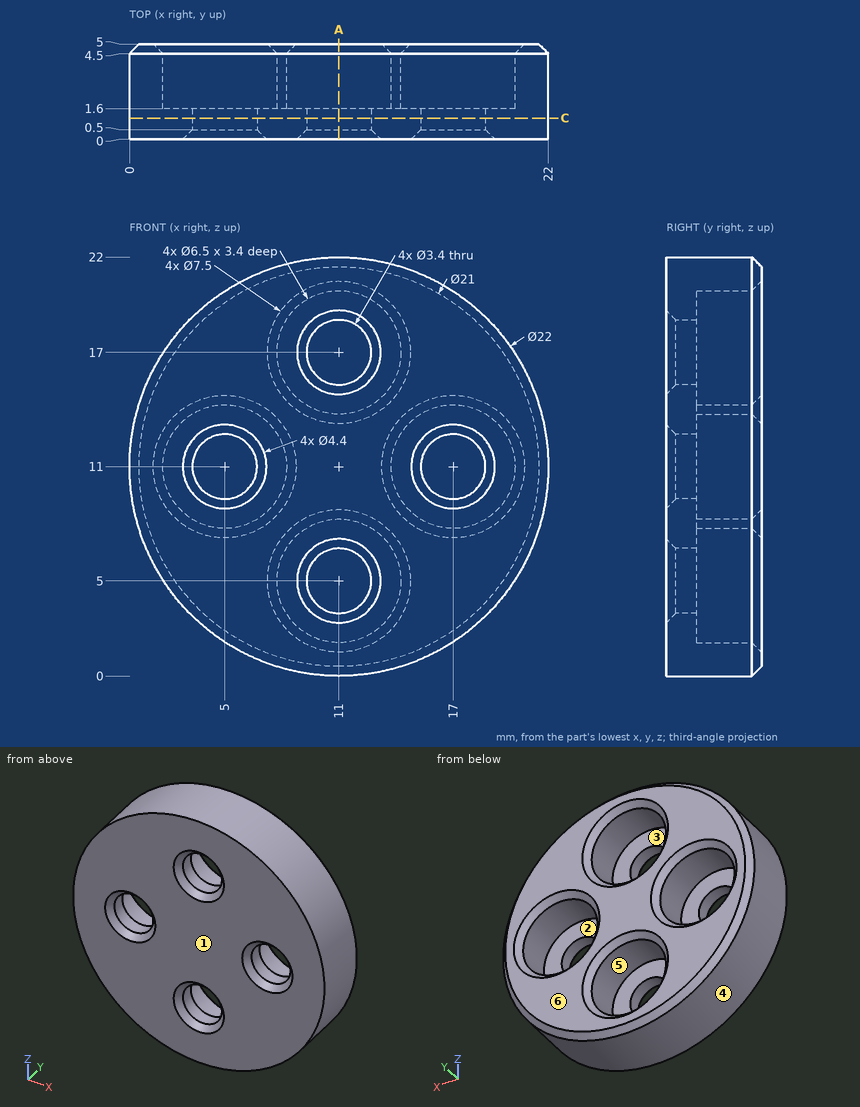
Check sheet for the drawn part. Datum: minimum x, y, z corner. Units: mm. A direction names the side the tool comes from. Give positions to 0.01 mm unless a question says otherwise; leave off trailing zeros. Write each loop counter-clockwise with the first axis right and the second up, starting at its lowest first coordinate (ties: lowest second). Pieces come first, ordered by that corner, then holes.
(1) Gauge pin test, flat ends, axial feed: pin 1 (6 mm diameter, centred on x = 11, z = 17, fed in from -Y); pin 2 (2.5 mm diameter, centred on x = 11, z = 17, fed in from -Y); pin 3 (4 mm diameter, centred on x = 11, z = 5, fed in from +Y); pin 4 (3 mm diameter, centred on y = 4, z = 16.5, fed in from +X). Record the tip position at first contact, or that the pin passes through.
(2) Cross-section at A-A (x = 11). State how many separate pieces and enclosed holes the cut face has, plus the area to 3 significant figures.
(3) Access from +Z, -Z, +X, -X, +Y, -Y to the whole of each face (thin tool, end or side, straight path). Record for the marked faces 5 and 6.
(4) Mould release check, pull along X, two halves, no side actions. Record for the marked faces 1, 2, 3 and 4: +X half, -X half, draft (parallel to the pull), parting line (faces both ways), or undercut.
(5) Cross-section at C-C (y = 1.1). Enter the section's corners in (x, z).
(6) Material ranges on line 1 (X direction, y = 3.6, z = 11); line 2 (Z direction, x = 11.5, y = 1.5); line 3 (Z direction, x = 12.5, y = 2.55), recorded low to high.
Worked out:
1. pin 1: stops at y = 0
1. pin 2: passes through
1. pin 3: stops at y = 1.6
1. pin 4: stops at x = 21.25
2. separate pieces: 3
2. enclosed holes: 0
2. area: 53.7 mm2
3. face 5: +Y
3. face 6: +Z, -Z, +X, -X, +Y
4. face 1: draft
4. face 2: undercut
4. face 3: undercut
4. face 4: parting line
5. outline: circle Ø22 at (11, 11); hole circle Ø3.4 at (5, 11); hole circle Ø3.4 at (11, 5); hole circle Ø3.4 at (11, 17); hole circle Ø3.4 at (17, 11)
6. line 1: x = 0 to 1.75, 8.25 to 13.75, 20.25 to 22
6. line 2: z = 0.01 to 3.38, 6.62 to 15.38, 18.62 to 21.99
6. line 3: z = 0.1 to 2.12, 7.88 to 14.12, 19.88 to 21.9
